Geometry check sheet. Reference: the model listing, model coordinates, mm. A direction names the side the tool comes from. Coordinates: 2 decimals unless noted, no trailing zeros. Write each loop counter-clockwise with the first axis right and the second up, starting at its lowest first coordinate (ties: lowest second). Pieces come first, ordered by that corner, then holes. Notation, with made-up numbers: M 17,70.25 L 59,70.25 A9 cw 59,79.25 Z; hole C 60.5,-3 d1. An arc over 180 degrees is marked long. Put each result on its own line as item: value. Start each with the question number.
1) Cross-section at C-C on z = -0.9. Record the cut outline in (x, y), plus the area to 3 significant figures.
2) Mould release check, pull along X, two halves, no side actions. Record for faces 1 (the flat face through (0, 20, 1)), 2 (the cylindrical face through (-20.5, -0.1, 0.5)), 3 (the flat face through (20, 0, -1)), 4 (the cylindrical face through (12, 0, 0)): released by +X, released by -X, zero draft, split by the parting line, or undercut.
3) Scan lines: line 1 along X through (y, z) = (0, 1); line 2 along Y through (x, z) = (-17.5, -0.2); line 3 along X through (y, z) = (1.5, 0.25). Record each from-to range of solid material in increasing order.
4) Cross-section at D-D on x = 15. Record the cut outline in (y, z).
5) Set-up check for faces 5 (the flat face through (-18, 5, -1)), 6 (the flat face through (15, 15, -1)), 7 (the flat face through (-5, 0, -1)), 8 (the flat face through (15, -15, -1)): record each of +Z, -Z, +X, -X, +Y, -Y from which the full face is reachable in a straight line by a thin tool's end or side.
6) Cross-section at A-A on x = -17.5. Record the cut outline in (y, z), plus the area to 3 significant figures.
7) Gauge pin test, flat ends, axial feed: pin 1 (1.6 mm diameter, centred on x = -12, z = -1, fed in from +Y); pin 2 (1.6 mm diameter, centred on x = 16, z = -1.5, fed in from -Y); pin 3 (1 mm diameter, centred on x = 12.5, z = -1.5, fed in from +Y). Record the tip position at first contact, or that the pin passes through.
8) Cross-section at B-B on y = 0. Record the cut outline in (x, z).
from build123d import *

# Parameters (mm, degrees)
F0_W     = 70
F0_H     = 40
F0_W_2   = 25
F0_H_2   = 10
F0_W_3   = 10
F0_H_3   = 30
F1_DEPTH = 3
F2_DEPTH = 2
F3_R     = 3
F4_R     = 3
F5_DEPTH = 25


with BuildPart() as f1:
    # F0 (on Top) → F1 (new body)
    with BuildSketch(Plane.XY):
        Rectangle(F0_W, F0_H)
        with Locations((-17.5, 0)):
            Rectangle(F0_W_2, F0_H_2, mode=Mode.SUBTRACT)
        with Locations((15, 0)):
            Rectangle(F0_W_3, F0_H_3, mode=Mode.SUBTRACT)
        with Locations((-17.5, 0)):
            Rectangle(F0_W_2, F0_H_2)
        with Locations((15, 0)):
            Rectangle(F0_W_3, F0_H_3)
    extrude(amount=F1_DEPTH)

    # F0 (on Top) → F2 (join)
    with BuildSketch(Plane.XY):
        with Locations((-17.5, 0)):
            Rectangle(F0_W_2, F0_H_2)
        with Locations((15, 0)):
            Rectangle(F0_W_3, F0_H_3)
    extrude(amount=-F2_DEPTH)

    # F3 (on face) + F4 (on face) → F5 (cut)
    with BuildSketch(Plane(origin=(0, 0, -2), x_dir=(1, 0, 0), z_dir=(0, 0, -1))):
        with Locations((-17.5, 0)):
            Circle(F3_R)
    with BuildSketch(Plane(origin=(0, 0, -2), x_dir=(1, 0, 0), z_dir=(0, 0, -1))):
        with Locations((15, 0)):
            Circle(F4_R)
    extrude(amount=-F5_DEPTH, mode=Mode.SUBTRACT)


solid = f1.part
Answer key:
1. outline: M -30,-5 L -5,-5 L -5,5 L -30,5 Z; M 10,-15 L 20,-15 L 20,15 L 10,15 Z; hole C -17.5,0 d6; hole C 15,0 d6
1. area: 493 mm²
2. face 1: zero draft
2. face 2: undercut
2. face 3: released by +X
2. face 4: undercut
3. line 1: x = -35 to -20.5, -14.5 to 12, 18 to 35
3. line 2: y = -5 to -3, 3 to 5
3. line 3: x = -35 to -20.1, -14.9 to 12.4, 17.6 to 35
4. outline: M -20,0 L -15,0 L -15,-2 L -3,-2 L -3,3 L -20,3 Z; M 3,-2 L 15,-2 L 15,0 L 20,0 L 20,3 L 3,3 Z
5. face 5: -Z, -X, +Y
5. face 6: -Z, +X, -X, +Y
5. face 7: -Z, +Y, -Y
5. face 8: -Z, +X, -X, -Y
6. outline: M -20,0 L -5,0 L -5,-2 L -3,-2 L -3,3 L -20,3 Z; M 3,-2 L 5,-2 L 5,0 L 20,0 L 20,3 L 3,3 Z
6. area: 110 mm²
7. pin 1: stops at y = 5
7. pin 2: stops at y = -15
7. pin 3: stops at y = 15
8. outline: M -35,0 L -30,0 L -30,-2 L -20.5,-2 L -20.5,3 L -35,3 Z; M -14.5,-2 L -5,-2 L -5,0 L 10,0 L 10,-2 L 12,-2 L 12,3 L -14.5,3 Z; M 18,-2 L 20,-2 L 20,0 L 35,0 L 35,3 L 18,3 Z
